Input: dimensioned drawing with shaded views. Units: mm. Origin: part minimum x, y, z. A direction names the side the tool comes from. Round coordinates to 2 decimals unless told otherwise and drop trailing zeros. Loops run counter-clockwise (first coordinate to the right, second up) from the corner with the lowest first, then second, coordinate; pieces in that order, holes last. Notation, with made-up numbers: M 54.5,28 L 104.5,28 A12 ccw 104.5,42 Z; hole C -10.75,89 d6. An arc over 180 degrees is marked long. Put each result on its own line as item: value. Start each with the question number.
1) Draft query along Y for the marked faces 1, 2, 3 and 4. Return one class per face: +Y half, -Y half, draft (parallel to the pull), parting line (faces both ways), or undercut.
2) Section D-D on x = 14. Output: boundary loops of the cut face in (y, z), plus the area to 3 significant figures.
3) Section C-C on z = 1. Output: boundary loops of the cut face in (x, y).
4) Reachability of the marked faces 5 and 6 from +Z, -Z, +X, -X, +Y, -Y: full face, straight path, thin tool, end or side. Return the list, or none.
5) Line query: probe 1 along Y at (x, z) = (5, 6); probe 2 along Y at (x, z) = (5, 2.25); probe 3 along Z at (x, y) = (25, 22.5). Output: solid intervals per line, ascending.
6) Pin query (flat end, axial travel): pin 1 (1 mm diameter, centred on x = 9.5, y = 38, fed in from -Z); pin 2 (1.5 mm diameter, centred on x = 14.5, z = 2, fed in from +Y); pin 3 (3 mm diameter, centred on x = 5, y = 46, fed in from -Z); pin 4 (0.8 mm diameter, centred on y = 29.5, z = 2.5, fed in from -X). Return the tip coordinate at first contact, or that it passes through.
7) Section B-B on y = 46. Output: boundary loops of the cut face in (x, z).
8) Section A-A on x = 5. Output: boundary loops of the cut face in (y, z).
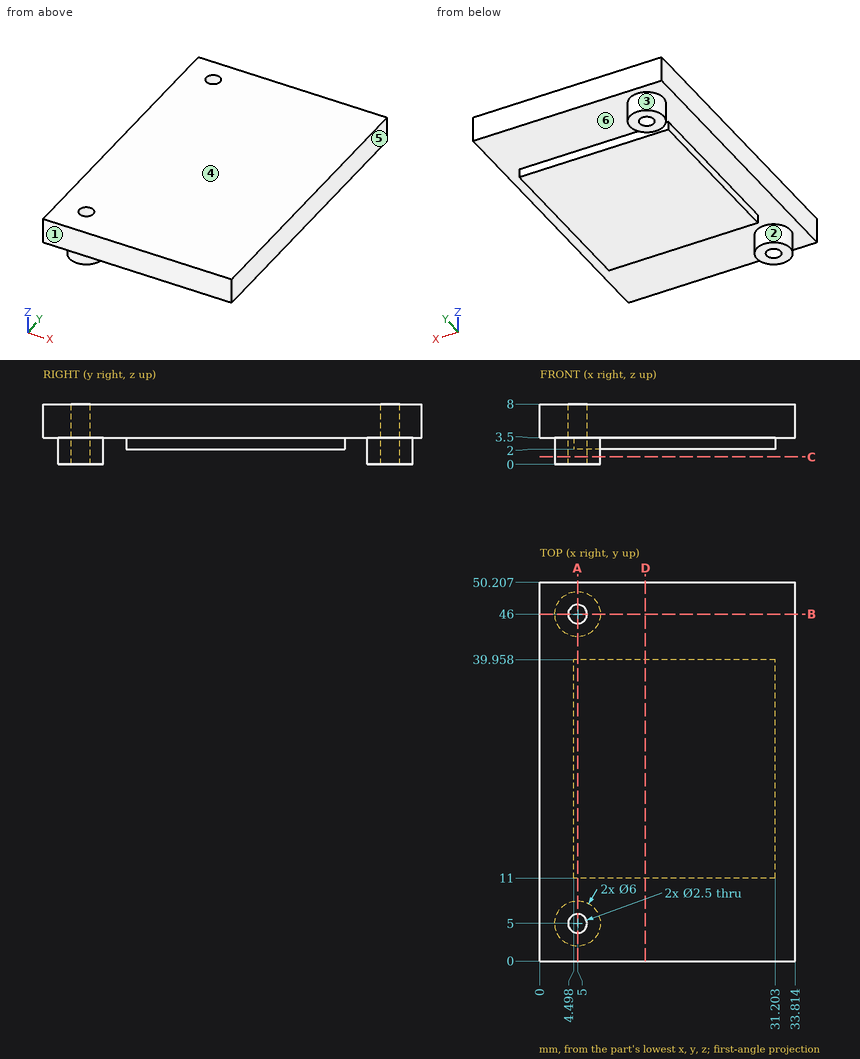
Geometry results:
1. face 1: -Y half
1. face 2: undercut
1. face 3: undercut
1. face 4: draft
2. outline: M 0,3.5 L 11,3.5 L 11,2 L 39.96,2 L 39.96,3.5 L 50.21,3.5 L 50.21,8 L 0,8 Z
2. area: 269 mm²
3. outline: C 5,5 d6; C 5,46 d6; hole C 5,5 d2.5; hole C 5,46 d2.5
4. face 5: +Z, -Z, +X, +Y, -Y
4. face 6: -Z
5. probe 1: y = 0 to 3.75, 6.25 to 44.75, 47.25 to 50.21
5. probe 2: y = 2 to 3.75, 6.25 to 8, 11 to 39.96, 43 to 44.75, 47.25 to 49
5. probe 3: z = 2 to 8
6. pin 1: stops at z = 2
6. pin 2: stops at y = 39.96
6. pin 3: stops at z = 0
6. pin 4: stops at x = 4.5
7. outline: M 0,3.5 L 2,3.5 L 2,0 L 3.75,0 L 3.75,8 L 0,8 Z; M 6.25,0 L 8,0 L 8,3.5 L 33.81,3.5 L 33.81,8 L 6.25,8 Z
8. outline: M 0,3.5 L 2,3.5 L 2,0 L 3.75,0 L 3.75,8 L 0,8 Z; M 6.25,0 L 8,0 L 8,3.5 L 11,3.5 L 11,2 L 39.96,2 L 39.96,3.5 L 43,3.5 L 43,0 L 44.75,0 L 44.75,8 L 6.25,8 Z; M 47.25,0 L 49,0 L 49,3.5 L 50.21,3.5 L 50.21,8 L 47.25,8 Z
